Here's how the part is built. I have some questions about the finished solid (model axes, mm). Round coordinates to 2 decimals unless told otherwise and drop trailing zeros. Write each loop counter-clockwise with the first axis right and the second up, starting at its lowest first coordinate (ties: lowest second). Pieces come first, ordered by that corner, then holes. Notation, with made-up numbers: M -1.5,45 L 46.5,45 A31 ccw 46.5,71 Z; hole C 62,83.5 d11. An arc over 180 degrees is marked long. Write item = value, one per line. Start each with the question number.
(1) I need wall thicknesses on line 1 along Y through (x, z) = (0, 1.7); line 2 along Y through (x, z) = (7, 0.2); line 3 along X through (y, z) = (-0.75, 2.6). Which ranges of each line are inside material? Lowest first, please.
(2) If we mould it in two halves opening along Y, with no side actions, what happens to faces 1 (the flat face through (4, 4, 3)), 2 (the cylindrical face through (1.617, -0.67, 1.479))? For each: released by +Y, released by -Y, zero draft, split by the parting line, or undercut.
(3) Will this pin go through, and if not, where does the flat tip stop? pin 1 Ø5 at (x, y) = (-2.5, 2.5) entering from -Z.
(4) I want a section at C-C (z = 2.6). Give the number of separate pieces and of enclosed holes in the cut face, and give its area (3 significant figures).
(5) I want a section at D-D (x = -2.25). List the corners of the cut face in (y, z) for me, and give its area (3 significant figures).
(6) I want a section at A-A (y = 8). List the corners of the cut face in (x, z) for me, and give its area (3 significant figures).
```python
from build123d import *

# Parameters (mm, degrees)
SKETCH_1_R      = 1.75
EXTRUDE_1_DEPTH = 3
FILLET_1_R      = 10


with BuildPart() as part:
    # Эскиз1 → Бобышка-Вытянуть1 (new body)
    with BuildSketch(Plane.XY):
        with BuildLine():
            ThreePointArc((10.061552813, 4), (11.181980515, 11.181980515), (4, 10.061552813))
            ThreePointArc((4, 10.061552813), (-3.181980515, 11.181980515), (-2.061552813, 4))
            ThreePointArc((-2.061552813, 4), (-3.181980515, -3.181980515), (4, -2.061552813))
            ThreePointArc((4, -2.061552813), (11.181980515, -3.181980515), (10.061552813, 4))
        make_face()
        Circle(SKETCH_1_R, mode=Mode.SUBTRACT)
        with Locations((8, 0)):
            Circle(SKETCH_1_R, mode=Mode.SUBTRACT)
        with Locations((0, 8)):
            Circle(SKETCH_1_R, mode=Mode.SUBTRACT)
        with Locations((8, 8)):
            Circle(SKETCH_1_R, mode=Mode.SUBTRACT)
    extrude(amount=EXTRUDE_1_DEPTH)

    # Скругление1
    fillet_1_edges = [part.edges().sort_by_distance(p)[0] for p in [
        (10.061552813, 4, 1.5),
        (4, -2.061552813, 1.5),
        (-2.061552813, 4, 1.5),
        (4, 10.061552813, 1.5),
    ]]
    fillet(fillet_1_edges, radius=FILLET_1_R)


solid = part.part
```
Returned:
q1.line_1 = -4.5 to -1.75, 1.75 to 6.25, 9.75 to 12.5
q1.line_2 = -4.39 to -1.44, 1.44 to 6.56, 9.44 to 12.39
q1.line_3 = -4.44 to -1.58, 1.58 to 6.42, 9.58 to 12.44
q2.face_1 = zero draft
q2.face_2 = undercut
q3.pin_1 = 0
q4.separate_pieces = 1
q4.enclosed_holes = 4
q4.area = 223 mm²
q5.outline = M -3.9,0 L 11.9,0 L 11.9,3 L -3.9,3 Z
q5.area = 47.4 mm²
q6.outline = M -4.5,0 L -1.75,0 L -1.75,3 L -4.5,3 Z; M 1.75,0 L 6.25,0 L 6.25,3 L 1.75,3 Z; M 9.75,0 L 12.5,0 L 12.5,3 L 9.75,3 Z
q6.area = 30.0 mm²
